Here's how the part is built. I have some questions about the finished solid (model axes, mm). Face numbers are marked on the shaded views. A direction names the side the tool comes from. Round coordinates to 2 decimals unless told otherwise and drop trailing zeros. Write each loop counter-clockwise with the first axis right and the second up, starting at its lowest first coordinate (ties: lowest second). Pieces come first, ordered by that corner, then holes. Notation, with made-up numbers: (77.25, 83) - (121.25, 83) arc R33 ccw to (121.25, 111) - close; hole circle Ø4 at (-32.5, 20). An arc over 180 degrees is marked (long way). Use one line per item in the form item = value. Start each with the question number.
1. I want a section at A-A, the plane z = -23. List the corners of the cut face in (x, y) for me, plus the area to 3 significant figures.
2. Will these pins go through, and if not, where does the flat tip stop? pin 1 (23 mm diameter, centred on x = -4.5, y = -8, fed in from +Z); pin 2 (8 mm diameter, centred on x = -14.5, y = -0.5, fed in from -Z).
3. We'd pull the mould along X, two halves only. Please class the marked faces 1, 2, 3 and 4: +X half, -X half, draft (parallel to the pull), parting line (faces both ways), or undercut.
4. I want a section at B-B, the plane y = -21. List the corners of the cut face in (x, z) for me, plus the area to 3 significant figures.
5. If I drill on line 1 along Y through (x, z) = (-13, -24); line 2 along Z through (x, y) = (8, 2), over which ranges is the centre line in solid material (lowest first)?
6. I want a section at D-D, the plane z = 39.5. List the corners of the cut face in (x, y) for me.
7. Which directions (+Z, -Z, +X, -X, +Y, -Y) give clear straight access to the entire face, cutting with the end or side of a thin tool? Please do the marked faces 5, 6 and 7.
8. I want a section at C-C, the plane x = -16. List the corners of the cut face in (y, z) for me.
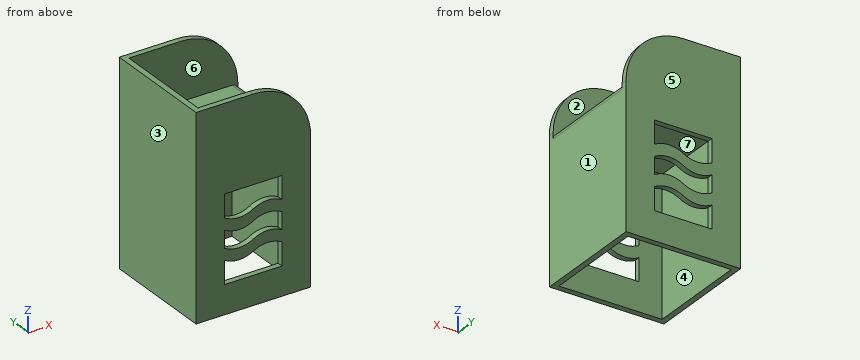
```python
from build123d import *

# Parameters (mm, degrees)
F0_W     = 50.8
F0_H     = 63.5
F1_DEPTH = 25.4
F2_T     = -2.54
F4_DEPTH = 25.4
F5_R     = 25.4
F6_R     = 2.54
F8_DEPTH = 50.8


with BuildPart() as f1:
    # F0 (on Right) → F1 (new body, symmetric)
    with BuildSketch(Plane.YZ):
        Rectangle(F0_W, F0_H)
        Polygon((12.7, -2.54), (12.7, -12.7), (-12.7, -12.7), (-12.7, -2.54), (-12.7, 2.54), (-12.7, 10.16), (-12.7, 15.24), (-12.7, 25.4), (12.7, 25.4), (12.7, 15.24), (12.7, 10.16), (12.7, 2.54), align=None, mode=Mode.SUBTRACT)
        with BuildLine():
            Line((-12.7, -12.7), (12.7, -12.7))
            Line((12.7, -12.7), (12.7, -2.54))
            ThreePointArc((12.7, -2.54), (6.35, -0.8385226281), (0, -2.54))
            ThreePointArc((0, -2.54), (-6.35, -4.2414773719), (-12.7, -2.54))
            Line((-12.7, -2.54), (-12.7, -12.7))
        make_face()
        with BuildLine():
            ThreePointArc((0, 15.24), (6.35, 16.9414773719), (12.7, 15.24))
            Line((12.7, 15.24), (12.7, 25.4))
            Line((12.7, 25.4), (-12.7, 25.4))
            Line((-12.7, 25.4), (-12.7, 15.24))
            ThreePointArc((-12.7, 15.24), (-6.35, 13.5385226281), (0, 15.24))
        make_face()
        with BuildLine():
            ThreePointArc((0, 2.54), (6.35, 4.2414773719), (12.7, 2.54))
            Line((12.7, 2.54), (12.7, 10.16))
            ThreePointArc((12.7, 10.16), (6.35, 11.8614773719), (0, 10.16))
            ThreePointArc((0, 10.16), (-6.35, 8.4585226281), (-12.7, 10.16))
            Line((-12.7, 10.16), (-12.7, 2.54))
            ThreePointArc((-12.7, 2.54), (-6.35, 0.8385226281), (0, 2.54))
        make_face()
        with BuildLine():
            ThreePointArc((0, 10.16), (6.35, 11.8614773719), (12.7, 10.16))
            Line((12.7, 10.16), (12.7, 15.24))
            ThreePointArc((12.7, 15.24), (6.35, 16.9414773719), (0, 15.24))
            ThreePointArc((0, 15.24), (-6.35, 13.5385226281), (-12.7, 15.24))
            Line((-12.7, 15.24), (-12.7, 10.16))
            ThreePointArc((-12.7, 10.16), (-6.35, 8.4585226281), (0, 10.16))
        make_face()
        with BuildLine():
            ThreePointArc((0, -2.54), (6.35, -0.8385226281), (12.7, -2.54))
            Line((12.7, -2.54), (12.7, 2.54))
            ThreePointArc((12.7, 2.54), (6.35, 4.2414773719), (0, 2.54))
            ThreePointArc((0, 2.54), (-6.35, 0.8385226281), (-12.7, 2.54))
            Line((-12.7, 2.54), (-12.7, -2.54))
            ThreePointArc((-12.7, -2.54), (-6.35, -4.2414773719), (0, -2.54))
        make_face()
    extrude(amount=F1_DEPTH, both=True)

    # F2
    f2_openings = [f1.faces().sort_by_distance(p)[0] for p in [
        (0, 0, -31.75),
    ]]
    offset(amount=F2_T, openings=f2_openings)

    # F3 (on face) → F4 (join)
    with BuildSketch(Plane.XY.offset(31.75)):
        Polygon((25.4, -25.4), (25.4, -22.86), (-22.86, -22.86), (-22.86, 22.86), (25.4, 22.86), (25.4, 25.4), (-25.4, 25.4), (-25.4, -25.4), align=None)
    extrude(amount=F4_DEPTH)

    # F5
    f5_edges = [f1.edges().sort_by_distance(p)[0] for p in [
        (25.4, -24.13, 57.15),
        (25.4, 24.13, 57.15),
    ]]
    fillet(f5_edges, radius=F5_R)

    # F6
    f6_edges = [f1.edges().sort_by_distance(p)[0] for p in [
        (25.4, 0, 31.75),
    ]]
    fillet(f6_edges, radius=F6_R)

    # F7 (on face) → F8 (cut)
    with BuildSketch(Plane.XZ.offset(25.4)):
        with BuildLine():
            Line((-12.7, 19.05), (-12.7, 8.89))
            ThreePointArc((-12.7, 8.89), (-6.35, 7.1885226281), (0, 8.89))
            ThreePointArc((0, 8.89), (6.35, 10.5914773719), (12.7, 8.89))
            Line((12.7, 8.89), (12.7, 19.05))
            Line((12.7, 19.05), (-12.7, 19.05))
        make_face()
        with BuildLine():
            Line((-12.7, 3.81), (-12.7, -3.81))
            ThreePointArc((-12.7, -3.81), (-6.35, -5.5114773719), (0, -3.81))
            ThreePointArc((0, -3.81), (6.35, -2.1085226281), (12.7, -3.81))
            Line((12.7, -3.81), (12.7, 3.81))
            ThreePointArc((12.7, 3.81), (6.35, 5.5114773719), (0, 3.81))
            ThreePointArc((0, 3.81), (-6.35, 2.1085226281), (-12.7, 3.81))
        make_face()
        with BuildLine():
            Line((-12.7, -8.89), (-12.7, -19.05))
            Line((-12.7, -19.05), (12.7, -19.05))
            Line((12.7, -19.05), (12.7, -8.89))
            ThreePointArc((12.7, -8.89), (6.35, -7.1885226281), (0, -8.89))
            ThreePointArc((0, -8.89), (-6.35, -10.5914773719), (-12.7, -8.89))
        make_face()
    extrude(amount=-F8_DEPTH, mode=Mode.SUBTRACT)


solid = f1.part
```
Model answer:
q1.outline = (-25.4, -25.4) - (25.4, -25.4) - (25.4, 25.4) - (-25.4, 25.4) - close; hole (-22.86, -22.86) - (22.86, -22.86) - (22.86, 22.86) - (-22.86, 22.86) - close
q1.area = 490 mm2
q2.pin_1 = 31.75
q2.pin_2 = 29.21
q3.face_1 = +X half
q3.face_2 = draft
q3.face_3 = -X half
q3.face_4 = undercut
q4.outline = (-25.4, -31.75) - (-22.86, -31.75) - (-22.86, 29.21) - (22.86, 29.21) - (22.86, -31.75) - (25.4, -31.75) - (25.4, 29.21) arc R2.54 ccw to (22.86, 31.75) - (-22.86, 31.75) - (-22.86, 57.15) - (-25.4, 57.15) - close
q4.area = 502 mm2
q5.line_1 = -25.4 to -22.86, 22.86 to 25.4
q5.line_2 = 29.21 to 31.75
q6.outline = (-25.4, -25.4) - (24.19, -25.4) - (24.19, -22.86) - (-22.86, -22.86) - (-22.86, 22.86) - (24.19, 22.86) - (24.19, 25.4) - (-25.4, 25.4) - close
q7.face_5 = +Z, -Z, +X, -X, +Y
q7.face_6 = +Z, +X
q7.face_7 = -Z
q8.outline = (-25.4, -31.75) - (-22.86, -31.75) - (-22.86, 29.21) - (22.86, 29.21) - (22.86, -31.75) - (25.4, -31.75) - (25.4, 57.15) - (22.86, 57.15) - (22.86, 31.75) - (-22.86, 31.75) - (-22.86, 57.15) - (-25.4, 57.15) - close
